from build123d import *

# Parameters (mm, degrees)
F1_DEPTH = 50.8
F0_R     = 76.2
F0_R_2   = 38.1
F2_DEPTH = 127


with BuildPart() as f1:
    # F0 (on Top) → F1 (new body)
    with BuildSketch(Plane.XY):
        with BuildLine():
            Line((-355.6, -508), (-97.9242677745, -508))
            ThreePointArc((-97.9242677745, -508), (-31.6872932017, -469.4709861755), (34.5496813712, -508))
            Line((34.5496813712, -508), (355.6, -508))
            ThreePointArc((355.6, -508), (373.5605122421, -500.5605122421), (381, -482.6))
            Line((381, -482.6), (381, -393.7))
            ThreePointArc((381, -393.7), (366.1210244843, -429.6210244843), (330.2, -444.5))
            Line((330.2, -444.5), (-330.2, -444.5))
            ThreePointArc((-330.2, -444.5), (-366.1210244843, -429.6210244843), (-381, -393.7))
            Line((-381, -393.7), (-381, -482.6))
            ThreePointArc((-381, -482.6), (-373.5605122421, -500.5605122421), (-355.6, -508))
        make_face()
    extrude(amount=F1_DEPTH)

    # F0 (on Top) → F2 (join)
    with BuildSketch(Plane.XY):
        with BuildLine():
            ThreePointArc((419.1, 520.7), (404.2210244843, 556.6210244843), (368.3, 571.5))
            Line((368.3, 571.5), (-419.1, 571.5))
            ThreePointArc((-419.1, 571.5), (-455.0210244843, 556.6210244843), (-469.9, 520.7))
            Line((-469.9, 520.7), (-469.9, 448.4929144382))
            Line((-469.9, 448.4929144382), (-469.9, -520.7))
            ThreePointArc((-469.9, -520.7), (-455.0210244843, -556.6210244843), (-419.1, -571.5))
            Line((-419.1, -571.5), (-103.3762187401, -571.5))
            ThreePointArc((-103.3762187401, -571.5), (-107.6079819524, -539.1526259812), (-97.9242677745, -508))
            Line((-97.9242677745, -508), (-355.6, -508))
            ThreePointArc((-355.6, -508), (-373.5605122421, -500.5605122421), (-381, -482.6))
            Line((-381, -482.6), (-381, -393.7))
            Line((-381, -393.7), (-381, 63.5))
            ThreePointArc((-381, 63.5), (-366.1210244843, 99.4210244843), (-330.2, 114.3))
            Line((-330.2, 114.3), (-304.8, 114.3))
            ThreePointArc((-304.8, 114.3), (-268.8789755157, 129.1789755157), (-254, 165.1))
            Line((-254, 165.1), (-254, 205.8778104236))
            ThreePointArc((-254, 205.8778104236), (-244.8700196616, 234.9337816068), (-220.7618322284, 253.5456407579))
            Line((-220.7618322284, 253.5456407579), (160.2381677716, 393.9140618106))
            ThreePointArc((160.2381677716, 393.9140618106), (206.8559711832, 387.9162511379), (228.6, 346.2462314763))
            Line((228.6, 346.2462314763), (228.6, 63.5))
            ThreePointArc((228.6, 63.5), (236.0394877579, 45.5394877579), (254, 38.1))
            Line((254, 38.1), (355.6, 38.1))
            ThreePointArc((355.6, 38.1), (373.5605122421, 30.6605122421), (381, 12.7))
            Line((381, 12.7), (381, -393.7))
            Line((381, -393.7), (381, -482.6))
            ThreePointArc((381, -482.6), (373.5605122421, -500.5605122421), (355.6, -508))
            Line((355.6, -508), (34.5496813712, -508))
            ThreePointArc((34.5496813712, -508), (41.9798550479, -526.1878840413), (44.5127067983, -545.6709861755))
            ThreePointArc((44.5127067983, -545.6709861755), (43.3764667828, -558.7809799584), (40.0016323368, -571.5))
            Line((40.0016323368, -571.5), (419.1, -571.5))
            ThreePointArc((419.1, -571.5), (455.0210244843, -556.6210244843), (469.9, -520.7))
            Line((469.9, -520.7), (469.9, 114.3))
            Line((469.9, 114.3), (419.1, 114.3))
            Line((419.1, 114.3), (419.1, 448.4929144382))
            Line((419.1, 448.4929144382), (419.1, 520.7))
        make_face()
        with BuildLine():
            ThreePointArc((-317.5, 448.4929144382), (-393.7, 372.2929144382), (-469.9, 448.4929144382))
            ThreePointArc((-469.9, 448.4929144382), (-393.7, 524.6929144382), (-317.5, 448.4929144382))
        make_face(mode=Mode.SUBTRACT)
        with Locations((342.9, 448.4929144382)):
            Circle(F0_R, mode=Mode.SUBTRACT)
        with BuildLine():
            ThreePointArc((-317.5, 448.4929144382), (-393.7, 524.6929144382), (-469.9, 448.4929144382))
            ThreePointArc((-469.9, 448.4929144382), (-393.7, 372.2929144382), (-317.5, 448.4929144382))
        make_face()
        with Locations((-393.7, 448.4929144382)):
            Circle(F0_R_2, mode=Mode.SUBTRACT)
        with Locations((342.9, 448.4929144382)):
            Circle(F0_R)
        with Locations((342.9, 448.4929144382)):
            Circle(F0_R_2, mode=Mode.SUBTRACT)
        with BuildLine():
            Line((-3.6788650977, -571.5), (40.0016323368, -571.5))
            ThreePointArc((40.0016323368, -571.5), (43.3764667828, -558.7809799584), (44.5127067983, -545.6709861755))
            ThreePointArc((44.5127067983, -545.6709861755), (41.9798550479, -526.1878840413), (34.5496813712, -508))
            Line((34.5496813712, -508), (-25.9858196586, -508))
            ThreePointArc((-25.9858196586, -508), (-2.8009976449, -520.8276383938), (6.4127067983, -545.6709861755))
            ThreePointArc((6.4127067983, -545.6709861755), (3.8002476455, -559.5362104658), (-3.6788650977, -571.5))
        make_face()
        with BuildLine():
            ThreePointArc((34.5496813712, -508), (-31.6872932017, -469.4709861755), (-97.9242677745, -508))
            Line((-97.9242677745, -508), (-37.3887667448, -508))
            ThreePointArc((-37.3887667448, -508), (-31.6872932017, -507.5709861755), (-25.9858196586, -508))
            Line((-25.9858196586, -508), (34.5496813712, -508))
        make_face()
        with BuildLine():
            ThreePointArc((-97.9242677745, -508), (-107.6079819524, -539.1526259812), (-103.3762187401, -571.5))
            Line((-103.3762187401, -571.5), (-59.6957213057, -571.5))
            ThreePointArc((-59.6957213057, -571.5), (-67.633807181, -533.0433128848), (-37.3887667448, -508))
            Line((-37.3887667448, -508), (-97.9242677745, -508))
        make_face()
        with BuildLine():
            Line((-59.6957213057, -571.5), (-103.3762187401, -571.5))
            ThreePointArc((-103.3762187401, -571.5), (-31.6872932017, -621.8709861755), (40.0016323368, -571.5))
            Line((40.0016323368, -571.5), (-3.6788650977, -571.5))
            ThreePointArc((-3.6788650977, -571.5), (-31.6872932017, -583.7709861755), (-59.6957213057, -571.5))
        make_face()
    extrude(amount=F2_DEPTH)


solid = f1.part
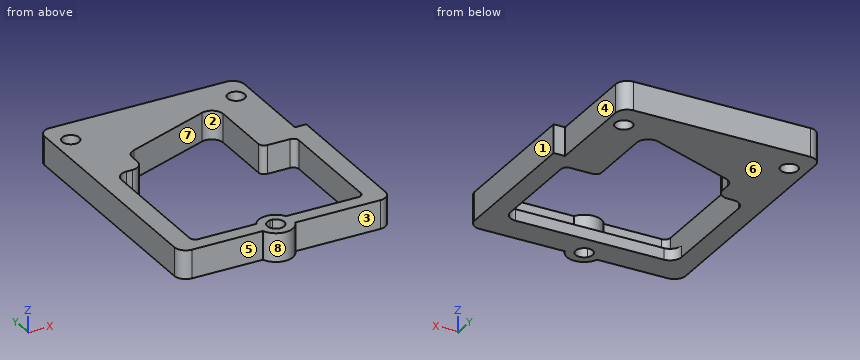
Input: part model. Units: mm. Frame: model coordinates. Face numbers are marked on the shaded views. A direction names the side the tool comes from. Round coordinates to 2 decimals unless told otherwise and drop trailing zeros. Order: outer loops, then holes, each group sorted by start corner. A loop starts at its lowest first (then second) coordinate and runs counter-clockwise, first axis right, second up. Notation, with made-up numbers: (86, 52.5) - (104, 52.5) arc R19 cw to (104, 75.5) - close; hole circle Ø10 at (64, -12.75). An arc over 180 degrees is marked (long way). Use a Markdown table: item, result.
1. Mould query, pull axis X, two halves, no side actions, for the marked faces 1, 2 and 3. Classes: +X half, -X half, draft (parallel to the pull), parting line (faces both ways), or undercut.
Evaluation:
| item | result |
|---|---|
| face 1 | +X half |
| face 2 | undercut |
| face 3 | draft |
2. Section A-A on y = -257. Return the cut outline in (x, z).
Evaluation:
| item | result |
|---|---|
| outline | (-469.9, 0) - (-381, 0) - (-381, 127) - (-469.9, 127) - close; (381, 0) - (469.9, 0) - (469.9, 127) - (381, 127) - close |
3. Section B-B on x = -393.7. Return the cut outline in (y, z).
Evaluation:
| item | result |
|---|---|
| outline | (-571.5, 0) - (410.39, 0) - (410.39, 127) - (-571.5, 127) - close; (486.59, 0) - (571.5, 0) - (571.5, 127) - (486.59, 127) - close |
4. First-contact query: pin 1 (7.5 mm diameter, centred on x = -321.5, z = 43.5, fed in from -Y); pin 2 (1 mm diameter, centred on x = 36, z = 64.5, fed in from -Y). Flat tips, straight axial feed; report the tip coordinate or a pass-through.
Evaluation:
| item | result |
|---|---|
| pin 1 | y = -571.5 |
| pin 2 | y = -581.62 |
5. Material intervals for probe 1 along Y at (x, z) = (342, 89); probe 2 along X at (y, z) = (-431, 105); probe 3 along X at (y, z) = (474, 107), sorted ascending.
Evaluation:
| item | result |
|---|---|
| probe 1 | -571.5 to -508, 38.1 to 410.4, 486.58 to 571.5 |
| probe 2 | -469.9 to -381, 381 to 469.9 |
| probe 3 | -469.9 to -422, -365.4 to 314.6, 371.2 to 419.1 |
6. Section C-C on x = 342.9. Return the cut outline in (y, z).
Evaluation:
| item | result |
|---|---|
| outline | (-571.5, 0) - (-442.89, 0) - (-442.89, 50.8) - (-508, 50.8) - (-508, 127) - (-571.5, 127) - close; (38.1, 0) - (410.39, 0) - (410.39, 127) - (38.1, 127) - close; (486.59, 0) - (571.5, 0) - (571.5, 127) - (486.59, 127) - close |
7. Section D-D on z = 28. State how many separate pieces and enclosed holes the cut face has, then the cut area to 4 significant figures.
Evaluation:
| item | result |
|---|---|
| separate pieces | 1 |
| enclosed holes | 4 |
| area | 524,500 mm^2 |
8. Access query for the marked faces 4, 5, 6, 7 and 8. Directions: +Z, -Z, +X, -X, +Y, -Y. A direction counts if a zero-diameter tool reaches every point of the face in a straight line with its end or side. Return the directions, or none.
Evaluation:
| item | result |
|---|---|
| face 4 | +Z, -Z, +X, +Y |
| face 5 | +Z, -Z, -X, -Y |
| face 6 | -Z, +X, -X, +Y, -Y |
| face 7 | +Z, -Z |
| face 8 | +Z, -Z, -Y |
